Can you work these out from the model? Positions are in its coordinate system, mm. Give positions to 0.01 mm unless a question says otherwise; leave off trailing zeros. Loops run counter-clockwise (first coordinate to the right, second up) from the corner with the lowest first, then second, coordinate; pieces in that order, holes last. Notation, with made-up numbers: (79, -12.5) -> (121, -12.5) arc R19 cw to (121, 1.5) -> close; hole circle Ø9 at (78.5, -7.5). An arc over 180 degrees is marked (long way). One line per question, with ' | ' between items.
from build123d import *

# Parameters (mm, degrees)
SKETCH1_R           = 19.685
SKETCH1_R_2         = 1.905
BOSS_EXTRUDE1_DEPTH = 4.572
SKETCH2_R           = 19.685
SKETCH2_R_2         = 17.78
BOSS_EXTRUDE2_DEPTH = 0.508


with BuildPart() as part:
    # Sketch1 → Boss-Extrude1 (new body)
    with BuildSketch(Plane.XY):
        with BuildLine():
            Line((-19.05, -31.75), (19.05, -31.75))
            ThreePointArc((19.05, -31.75), (28.030256121, -28.030256121), (31.75, -19.05))
            Line((31.75, -19.05), (31.75, 19.05))
            ThreePointArc((31.75, 19.05), (28.030256121, 28.030256121), (19.05, 31.75))
            Line((19.05, 31.75), (-19.05, 31.75))
            ThreePointArc((-19.05, 31.75), (-28.030256121, 28.030256121), (-31.75, 19.05))
            Line((-31.75, 19.05), (-31.75, -19.05))
            ThreePointArc((-31.75, -19.05), (-28.030256121, -28.030256121), (-19.05, -31.75))
        make_face()
        Circle(SKETCH1_R, mode=Mode.SUBTRACT)
        with Locations((-23.540128061, 23.540128061)):
            Circle(SKETCH1_R_2, mode=Mode.SUBTRACT)
        with Locations((23.540128061, 23.540128061)):
            Circle(SKETCH1_R_2, mode=Mode.SUBTRACT)
        with Locations((23.540128061, -23.540128061)):
            Circle(SKETCH1_R_2, mode=Mode.SUBTRACT)
        with Locations((-23.540128061, -23.540128061)):
            Circle(SKETCH1_R_2, mode=Mode.SUBTRACT)
    extrude(amount=BOSS_EXTRUDE1_DEPTH)

    # Sketch2 → Boss-Extrude2 (add)
    with BuildSketch(Plane.XY.offset(4.572)):
        Circle(SKETCH2_R)
        Circle(SKETCH2_R_2, mode=Mode.SUBTRACT)
    extrude(amount=-BOSS_EXTRUDE2_DEPTH)


solid = part.part
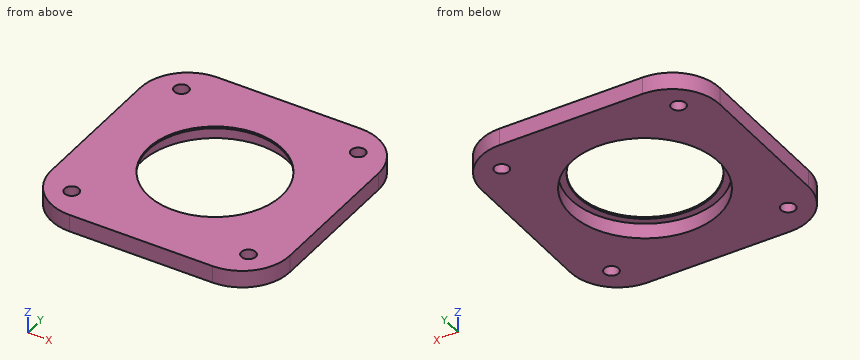
Q1. If I drill on probe 1 along X at (y, z) = (22, 1.2); probe 2 along X at (y, z) = (-23, 2.6); probe 3 along Y at (x, z) = (23.5, 2.7), over which ranges is the centre line in solid material (lowest first)? Write a range as from..to.
Entries:
probe 1: -31.4..-24.66, -22.42..22.42, 24.66..31.4 | probe 2: -31.12..-25.37, -21.71..21.71, 25.37..31.12 | probe 3: -30.94..-25.44, -21.64..21.64, 25.44..30.94
Q2. If we section it at A-A (x = 0): Write out the boundary of the cut face in (y, z) (3 decimals).
Entries:
outline: (-31.75, 0) -> (-19.685, 0) -> (-19.685, 4.064) -> (-17.78, 4.064) -> (-17.78, 4.572) -> (-31.75, 4.572) -> close; (17.78, 4.064) -> (19.685, 4.064) -> (19.685, 0) -> (31.75, 0) -> (31.75, 4.572) -> (17.78, 4.572) -> close
Q3. If we section it at C-C (z = 2.9): Write out the boundary of the cut face in (x, y) (3 decimals), plus the area to 3 significant figures.
Entries:
outline: (-31.75, -19.05) arc R12.7 ccw to (-19.05, -31.75) -> (19.05, -31.75) arc R12.7 ccw to (31.75, -19.05) -> (31.75, 19.05) arc R12.7 ccw to (19.05, 31.75) -> (-19.05, 31.75) arc R12.7 ccw to (-31.75, 19.05) -> close; hole circle Ø3.81 at (-23.54, -23.54); hole circle Ø3.81 at (-23.54, 23.54); hole circle Ø39.37 at (0, 0); hole circle Ø3.81 at (23.54, -23.54); hole circle Ø3.81 at (23.54, 23.54) | area: 2,630 mm²
Q4. For pin 1 Ø8 at (x, y) = (-11, 23) entering from -Z, with a flat end and sliding along its axis, tell me the tip position at first contact or that it passes through.
Entries:
pin 1: z = 0
